Geometry check sheet. Reference: the model listing, model coordinates, mm. A direction names the side the tool comes from. Coordinates: 2 decimals unless noted, no trailing zeros. Loops run counter-clockwise (first coordinate to the right, second up) from the corner with the lowest first, then second, coordinate; pieces in that order, holes last. Notation, with made-up numbers: (9, -35) - (46, -35) arc R33 ccw to (46, 3) - close; hole circle Ø4 at (-16.75, -19.75). An arc over 180 degrees is marked (long way). One line per item, written item: value.
from build123d import *

# Parameters (mm, degrees)
F0_W      = 63.5
F0_H      = 12.7
F1_DEPTH  = 88.9
F2_W      = 12.7
F2_H      = 50.8
F3_DEPTH  = 44.45
F1_FACE_W = 88.9
F1_FACE_H = 12.7
F4_DEPTH  = 12.7
F5_DEPTH  = 33.02
F6_W      = 12.7
F6_H      = 50.8
F7_DEPTH  = 44.45
F8_DEPTH  = 44.45


with BuildPart() as f1:
    # F0 (on Right) → F1 (new body)
    with BuildSketch(Plane.YZ):
        Rectangle(F0_W, F0_H)
    extrude(amount=F1_DEPTH)

    # F2 (on Front) → F3 (join)
    with BuildSketch(Plane.XZ):
        with Locations((-6.35, 18.538677)):
            Rectangle(F2_W, F2_H)
    extrude(amount=F3_DEPTH)

    # F1_face (on face) → F4 (join)
    with BuildSketch(Plane(origin=(44.45, -31.75, 0), x_dir=(1, 0, 0), z_dir=(0, -1, 0))):
        Rectangle(F1_FACE_W, F1_FACE_H)
    extrude(amount=F4_DEPTH)

    # F3_face (on face) → F5 (join)
    with BuildSketch(Plane(origin=(-6.35, 0, 18.538677), x_dir=(1, 0, 0), z_dir=(0, 1, 0))):
        Polygon((6.35, 24.888677), (6.35, 25.4), (-6.35, 25.4), (-6.35, -25.4), (6.35, -25.4), (6.35, 12.188677), align=None)
    extrude(amount=F5_DEPTH)

    # F6 (on Front) → F7 (join)
    with BuildSketch(Plane.XZ):
        with Locations((82.592454, 19.003852)):
            Rectangle(F6_W, F6_H)
    extrude(amount=F7_DEPTH)

    # F7_face (on face) → F8 (join)
    with BuildSketch(Plane(origin=(82.599499, 0, 25.310266), x_dir=(1, 0, 0), z_dir=(0, 1, 0))):
        Polygon((-6.357044, -19.093586), (6.342956, -19.093586), (6.342956, 31.706414), (-6.357044, 31.706414), (-6.357044, 31.660266), (6.300501, 31.660266), (6.300501, 18.960266), (-6.357044, 18.960266), align=None)
    extrude(amount=F8_DEPTH)


solid = f1.part
(1) Cross-section at D-D on x = 25.5. Record the cut outline in (y, z).
Reply:
outline: (-44.45, -6.35) - (31.75, -6.35) - (31.75, 6.35) - (-44.45, 6.35) - close
(2) Access from +Z, -Z, +X, -X, +Y, -Y to the whole of each face (thin tool, end or side, straight path). Record for faces 1 (the face through (-6, -6, 43.939)), 2 (the face through (38, -6, 6.35)), 3 (the face through (-6, 33.02, 18)).
Reply:
face 1: +Z, -X, +Y, -Y
face 2: +Z, +Y, -Y
face 3: +Z, -Z, -X, +Y
(3) Material ranges on probe 1 along X at (y, z) = (11.5, 29.5); probe 2 along Z at (x, y) = (54, 12), recorded low to high. Write a range as from..to.
Reply:
probe 1: -12.7..0, 76.24..88.94
probe 2: -6.35..6.35
(4) Cross-section at B-B on y = 39. Record the cut outline in (x, z), and give its area (3 significant figures).
Reply:
outline: (76.24, -6.4) - (88.94, -6.4) - (88.94, 44.4) - (76.24, 44.4) - (76.24, 6.35) - (88.9, 6.35) - (88.9, -6.35) - (76.24, -6.35) - close
area: 484 mm2
(5) Go/stop test with flat-tipped pins: pin 1 Ø3 at (x, y) = (23, -4.5) entering from +Z; pin 2 Ø14 at (x, y) = (82, 15) entering from -Z; pin 3 Ø6.5 at (x, z) = (-6, 16.5) entering from +Y. Record where each tip stops, or that it passes through.
Reply:
pin 1: z = 6.35
pin 2: z = -6.4
pin 3: y = 33.02
